Job drawing, mm, ordinate dimensions from the low corner. One solid piece. Coordinates: 2 decimals unless noted, no trailing zeros. Write each loop counter-clockwise with the first axis right and the second up, starting at its lowest first coordinate (ties: lowest second). Pieces come first, ordered by that corner, then holes. Notation, with made-up numbers: (35.5, 11) - (47.5, 11) arc R13 ccw to (47.5, 16) - close; hole circle Ø2 at (-25.75, -26.5). An arc over 180 degrees is marked (long way). Put each result on its own line as item: value. Start each with the question number.
1. Drill centre lines: L1, parallel to Y at x = 5, z = 106 (1 decimal); L2, parallel to X at y = 4.25, z = 81; L3, parallel to X at y = 6.5, z = 64.5 (1 decimal). Where is each one in solid material? Low to high. Write a range as from..to.
2. Saw through at A-A, the plane x = 1.25. Write the cut outline in (y, z) (1 decimal), plus the area to 3 significant figures.
3. Saw through at B-B, the plane z = 10. Write the cut outline in (x, y) (1 decimal).
4. Saw through at C-C, the plane y = 8. Write the cut outline in (x, z) (1 decimal).
5. Saw through at D-D, the plane z = 84. Write the cut outline in (x, y) (1 decimal).
6. Drop flat-ended pins along their axis: P1, Ø3, axis at x = 4.76, y = 4.76, coming from the -Z side; P2, Ø1, axis at y = 8.5, z = 40, coming from the +X side (1 decimal); P3, Ø2.5, axis at x = 4.76, y = 4.76, coming from the -Z side. Give the stop position or say it passes through.
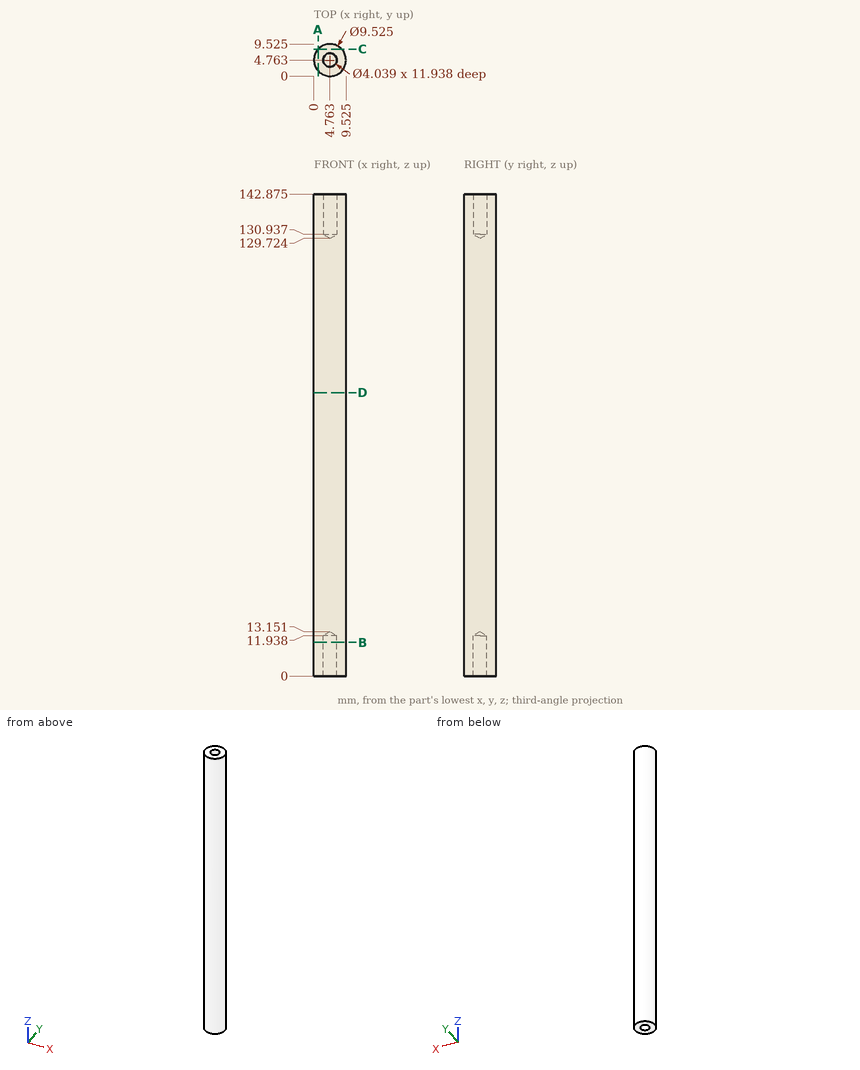
Final values:
1. L1: y = 0..9.5
1. L2: x = 0.03..9.5
1. L3: x = 0.3..9.2
2. outline: (1.5, 0) - (8, 0) - (8, 142.9) - (1.5, 142.9) - close
2. area: 919 mm²
3. outline: circle Ø9.5 at (4.8, 4.8); hole circle Ø4 at (4.8, 4.8)
4. outline: (1.3, 0) - (8.3, 0) - (8.3, 142.9) - (1.3, 142.9) - close
5. outline: circle Ø9.5 at (4.8, 4.8)
6. P1: stops at z = 12.25
6. P2: stops at x = 8.3
6. P3: stops at z = 12.4
